Design review of the part built by this model. Coordinates are the model's own, in mm. Face numbers are marked on the shaded views. A direction names the side the tool comes from. Coordinates: 2 decimals unless noted, no trailing zeros. Loops run counter-clockwise (first coordinate to the right, second up) from the corner with the lowest first, then second, coordinate; pieces in that order, holes last.
Q1. Machinability: for the marked faces 4 and 5, which of the approach directions +Z, -Z, +X, -X, +Y, -Y give a long, thin tool a straight path to every point of the face, cutting with its end or side? Answer none if there is none.
Q2. Add section C-C on z = 7. Give the boundary of the cut face in (x, y), and give its area (3 significant figures).
Q3. Wall thickness on probe 1 along Y at (x, z) = (0, 0.85); probe 2 along Y at (x, z) = (0, 5.25); probe 3 along Y at (x, z) = (-5, 0.75) (3 decimals): over which ranges is each line inside the solid? List them lowest first.
Q4. Add section D-D on y = -7.5. Give the boundary of the cut face in (x, z).
Q5. Draft analysis for pull direction Y (two halves, no side actions). For the marked faces 1, 2 and 3, state which applies: released by +Y, released by -Y, zero draft, split by the parting line, or undercut.
Q6. Add section A-A on y = 0. Give the boundary of the cut face in (x, z), and give its area (3 significant figures).
Q7. For P1, Ø5, axis at y = 6, z = 1, coming from the +X side; P2, Ø5, axis at x = -4.5, z = 4.5, coming from the -Y side; P3, Ø4, axis at x = -7.5, z = 3, coming from the -Y side, all flat-tipped, find the tip position at first contact; note any pin that passes through.
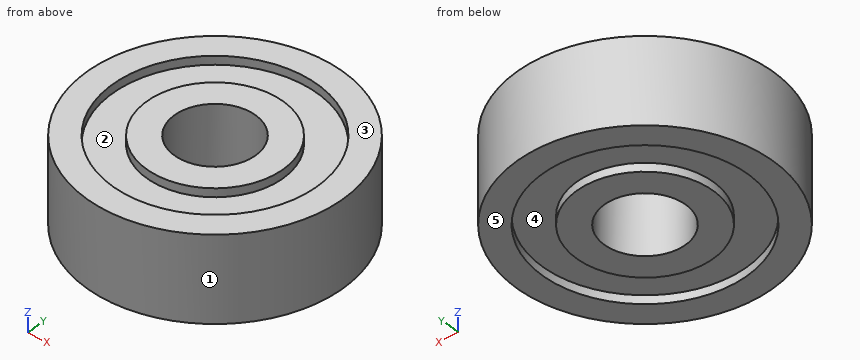
```python
from build123d import *

# Parameters (mm, degrees)
SKETCH1_R           = 15
SKETCH1_R_2         = 4.75
BOSS_EXTRUDE1_DEPTH = 10
SKETCH2_R           = 12
SKETCH2_R_2         = 8
CUT_EXTRUDE1_DEPTH  = 1
SKETCH4_R           = 12
SKETCH4_R_2         = 8
CUT_EXTRUDE2_DEPTH  = 1


with BuildPart() as part:
    # Sketch1 → Boss-Extrude1 (new body)
    with BuildSketch(Plane.XY):
        Circle(SKETCH1_R)
        Circle(SKETCH1_R_2, mode=Mode.SUBTRACT)
    extrude(amount=BOSS_EXTRUDE1_DEPTH)

    # Sketch2 → Cut-Extrude1 (cut)
    with BuildSketch(Plane.XY):
        Circle(SKETCH2_R)
        Circle(SKETCH2_R_2, mode=Mode.SUBTRACT)
    extrude(amount=CUT_EXTRUDE1_DEPTH, mode=Mode.SUBTRACT)

    # Sketch4 → Cut-Extrude2 (cut)
    with BuildSketch(Plane.XY.offset(10)):
        Circle(SKETCH4_R)
        Circle(SKETCH4_R_2, mode=Mode.SUBTRACT)
    extrude(amount=-CUT_EXTRUDE2_DEPTH, mode=Mode.SUBTRACT)


solid = part.part
```
Entries:
1. face 4: -Z
1. face 5: -Z, +X, -X, +Y, -Y
2. outline: circle Ø30 at (0, 0); hole circle Ø9.5 at (0, 0)
2. area: 636 mm2
3. probe 1: y = -15 to -12, -8 to -4.75, 4.75 to 8, 12 to 15
3. probe 2: y = -15 to -4.75, 4.75 to 15
3. probe 3: y = -14.142 to -10.909, -6.245 to 6.245, 10.909 to 14.142
4. outline: (-12.99, 0) - (-9.37, 0) - (-9.37, 1) - (-2.78, 1) - (-2.78, 0) - (2.78, 0) - (2.78, 1) - (9.37, 1) - (9.37, 0) - (12.99, 0) - (12.99, 10) - (9.37, 10) - (9.37, 9) - (2.78, 9) - (2.78, 10) - (-2.78, 10) - (-2.78, 9) - (-9.37, 9) - (-9.37, 10) - (-12.99, 10) - close
5. face 1: split by the parting line
5. face 2: undercut
5. face 3: zero draft
6. outline: (-15, 0) - (-12, 0) - (-12, 1) - (-8, 1) - (-8, 0) - (-4.75, 0) - (-4.75, 10) - (-8, 10) - (-8, 9) - (-12, 9) - (-12, 10) - (-15, 10) - close; (4.75, 0) - (8, 0) - (8, 1) - (12, 1) - (12, 0) - (15, 0) - (15, 10) - (12, 10) - (12, 9) - (8, 9) - (8, 10) - (4.75, 10) - close
6. area: 189 mm2
7. P1: stops at x = 14.59
7. P2: stops at y = -14.87
7. P3: stops at y = -13.96
